Part model, mm, in its own coordinate system. A direction names the side the tool comes from. Coordinates: 2 decimals unless noted, no trailing zeros. Order: outer loops, then holes, each group sorted by start corner. A loop starts at its lowest first (then second) coordinate and runs counter-clockwise, first axis right, second up.
1) Wall check: L1, parallel to X at y = -125, z = 0.75; L2, parallel to X at y = 155, z = 0.8; L3, parallel to X at y = 124, z = 0.35. Give the ranges that are in metal, low to high.
2) Cut at B-B (x = 37). List the corners of the cut face in (y, z).
3) Tool access for faces 1 (the cylindrical face through (0, 88, 1)), 2 (the cylindrical face through (124.719, 160.594, 0.749)): list every direction of +Z, -Z, +X, -X, +Y, -Y with a clear straight run to the whole face (end or side of a thin tool).
4) Cut at C-C (y = -78.5). List the corners of the cut face in (x, z).
5) Pin check, flat tips, straight feed: pin 1 Ø0.5 at (y, z) = (120.5, 0.5) entering from +X; pin 2 Ø0.5 at (y, z) = (53.5, 1) entering from -X. Stop position of each tip, or through.
6) Cut at A-A (y = 124.5). List the corners of the cut face in (x, z).
7) Cut at D-D (z = 0.5). Give the number of separate pieces and of enclosed holes in the cut face, and give its area (3 significant figures).
```python
from build123d import *

# Parameters (mm, degrees)
SKETCH1_W          = 254
SKETCH1_H          = 326
BASE_FLANGE1_DEPTH = 1.51892
SKETCH6_R          = 2.5
SKETCH6_W          = 1.5
SKETCH6_H          = 4
SKETCH6_W_2        = 35
SKETCH6_H_2        = 40
CUT_EXTRUDE1_DEPTH = 10
CUT_EXTRUDE2_DEPTH = 10


# Sheet-metal steps are written as plain solids
with BuildPart() as part:
    # Sketch1 → Base-Flange1 (new body)
    with BuildSketch(Plane.XY):
        Rectangle(SKETCH1_W, SKETCH1_H)
    extrude(amount=BASE_FLANGE1_DEPTH)

    # Sketch6 → Cut-Extrude1 (cut)
    with BuildSketch(Plane(origin=(0, 0, 0), x_dir=(-1, 0, 0), z_dir=(0, 0, -1))):
        with BuildLine():
            ThreePointArc((-124.99999998, 135), (-126.414213542, 135.585786438), (-126.99999998, 137))
            Line((-127, 137), (-127, -137))
            ThreePointArc((-126.99999998, -137), (-126.414213542, -135.585786438), (-124.99999998, -135))
            Line((-124.99999998, -135), (-119, -135))
            Line((-119, -135), (-119, -145))
            Line((-119, -145), (-115, -145))
            Line((-115, -145), (-115, -135))
            Line((-115, -135), (-109, -135))
            ThreePointArc((-109, -135), (-107.585786438, -134.414213562), (-107, -133))
            Line((-107, -133), (-107, 133))
            ThreePointArc((-107, 133), (-107.585786438, 134.414213562), (-109, 135))
            Line((-109, 135), (-115, 135))
            Line((-115, 135), (-115, 145))
            Line((-115, 145), (-119, 145))
            Line((-119, 145), (-119, 135))
            Line((-119, 135), (-124.99999998, 135))
        make_face()
        with Locations((-119, 155)):
            Circle(SKETCH6_R)
        with BuildLine():
            ThreePointArc((-126.99999998, 155), (-124.656854247, 160.656854252), (-119, 163))
            Line((-119, 163), (-127, 163))
            Line((-127, 163), (-127, 155))
        make_face()
        with Locations((-121.75, 140)):
            Rectangle(SKETCH6_W, SKETCH6_H)
        with Locations((-112.25, 140)):
            Rectangle(SKETCH6_W, SKETCH6_H)
        with Locations((-69.5, 127)):
            Rectangle(SKETCH6_W_2, SKETCH6_H_2)
        with BuildLine():
            Line((127, -137), (127, 137))
            ThreePointArc((127, 137), (126.414213562, 135.585786438), (125, 135))
            Line((125, 135), (119, 135))
            Line((119, 135), (119, 145))
            Line((119, 145), (115, 145))
            Line((115, 145), (115, 135))
            Line((115, 135), (109, 135))
            ThreePointArc((109, 135), (107.585786438, 134.414213562), (107, 133))
            Line((107, 133), (107, -133))
            ThreePointArc((107, -133), (107.585786438, -134.414213562), (109, -135))
            Line((109, -135), (115, -135))
            Line((115, -135), (115, -145))
            Line((115, -145), (119, -145))
            Line((119, -145), (119, -135))
            Line((119, -135), (125, -135))
            ThreePointArc((125, -135), (126.414213562, -135.585786438), (127, -137))
        make_face()
        with Locations((121.75, 140)):
            Rectangle(SKETCH6_W, SKETCH6_H)
        with Locations((112.25, 140)):
            Rectangle(SKETCH6_W, SKETCH6_H)
        with Locations((119, 155)):
            Circle(SKETCH6_R)
        with Locations((69.5, 127)):
            Rectangle(SKETCH6_W_2, SKETCH6_H_2)
        with BuildLine():
            ThreePointArc((119, 163), (124.656854249, 160.656854249), (127, 155))
            Line((127, 155), (127, 163))
            Line((127, 163), (119, 163))
        make_face()
        with BuildLine():
            ThreePointArc((-10, 113), (-6.464466094, 114.464466094), (-5, 118))
            Line((-5, 118), (-5, 142))
            ThreePointArc((-5, 142), (0, 147), (5, 142))
            Line((5, 142), (5, 118))
            ThreePointArc((5, 118), (6.464466094, 114.464466094), (10, 113))
            Line((10, 113), (12.5, 113))
            Line((12.5, 113), (12.5, 100.5))
            ThreePointArc((12.5, 100.5), (0, 88), (-12.5, 100.5))
            Line((-12.5, 100.5), (-12.5, 113))
            Line((-12.5, 113), (-10, 113))
        make_face()
        with Locations((-69.5, -127)):
            Rectangle(SKETCH6_W_2, SKETCH6_H_2)
        with Locations((-119, -155)):
            Circle(SKETCH6_R)
        with BuildLine():
            Line((-127, -163), (-119, -163))
            ThreePointArc((-119, -163), (-124.656854232, -160.656854238), (-126.99999998, -155))
            Line((-127, -155), (-127, -163))
        make_face()
        with Locations((-121.75, -140)):
            Rectangle(SKETCH6_W, SKETCH6_H)
        with Locations((-112.25, -140)):
            Rectangle(SKETCH6_W, SKETCH6_H)
        with Locations((69.5, -127)):
            Rectangle(SKETCH6_W_2, SKETCH6_H_2)
        with Locations((112.25, -140)):
            Rectangle(SKETCH6_W, SKETCH6_H)
        with Locations((121.75, -140)):
            Rectangle(SKETCH6_W, SKETCH6_H)
        with Locations((119, -155)):
            Circle(SKETCH6_R)
        with BuildLine():
            Line((127, -163), (127, -155))
            ThreePointArc((127, -155), (124.656854249, -160.656854249), (119, -163))
            Line((119, -163), (127, -163))
        make_face()
    extrude(amount=-CUT_EXTRUDE1_DEPTH, mode=Mode.SUBTRACT)

    # Sketch7 → Cut-Extrude2 (cut)
    with BuildSketch(Plane(origin=(0, 0, 0), x_dir=(-1, 0, 0), z_dir=(0, 0, -1))):
        Polygon((85, -70.857864376), (85, 70.857864376), (14.142135624, 0), align=None)
        Polygon((0, 14.142135624), (70.857864376, 85), (-70.857864376, 85), align=None)
        Polygon((-85, -70.857864376), (-14.142135624, 0), (-85, 70.857864376), align=None)
        Polygon((70.857864376, -85), (0, -14.142135624), (-70.857864376, -85), align=None)
    extrude(amount=-CUT_EXTRUDE2_DEPTH, mode=Mode.SUBTRACT)


solid = part.part
```
Geometry check:
1. L1: x = -107 to -87, -52 to 52, 87 to 107
1. L2: x = -127 to -121.5, -116.5 to 116.5, 121.5 to 127
1. L3: x = -107 to -87, -52 to -5, 5 to 52, 87 to 107
2. outline: (-163, 0) - (-85, 0) - (-85, 1.52) - (-163, 1.52) - close; (-51.14, 0) - (-22.86, 0) - (-22.86, 1.52) - (-51.14, 1.52) - close; (22.86, 0) - (51.14, 0) - (51.14, 1.52) - (22.86, 1.52) - close; (85, 0) - (163, 0) - (163, 1.52) - (85, 1.52) - close
3. face 1: +Z, -Z
3. face 2: +Z, -Z, +X, +Y
4. outline: (-107, 0) - (-64.36, 0) - (-64.36, 1.52) - (-107, 1.52) - close; (64.36, 0) - (107, 0) - (107, 1.52) - (64.36, 1.52) - close
5. pin 1: stops at x = 107
5. pin 2: stops at x = -107
6. outline: (-107, 0) - (-87, 0) - (-87, 1.52) - (-107, 1.52) - close; (-52, 0) - (-5, 0) - (-5, 1.52) - (-52, 1.52) - close; (5, 0) - (52, 0) - (52, 1.52) - (5, 1.52) - close; (87, 0) - (107, 0) - (107, 1.52) - (87, 1.52) - close
7. separate pieces: 1
7. enclosed holes: 21
7. area: 45,100 mm2
